Can you work these out from the model? Positions are in its coordinate system, mm. A direction names the side the tool comes from. Give positions to 0.01 mm unless a question says otherwise; leave off trailing zeros. Write each loop counter-clockwise with the first axis right and the second up, starting at its lowest first coordinate (ties: lowest second). Pieces come first, ordered by that corner, then holes.
from build123d import *

# Parameters (mm, degrees)
SKETCH_1_W          = 45
SKETCH_1_H          = 26
EXTRUDE_1_DEPTH     = 18
SKETCH_2_W          = 47
SKETCH_2_H          = 28
EXTRUDE_2_DEPTH     = 2
SKETCH_3_W          = 39
SKETCH_3_H          = 20
CUT_EXTRUDE_2_DEPTH = 2
CHAMFER_1_SIZE      = 2


with BuildPart() as part:
    # 草图1 → 凸台-拉伸1 (new body)
    with BuildSketch(Plane(origin=(0, 0, 0), x_dir=(1, 0, 0), z_dir=(0, 1, 0))):
        Rectangle(SKETCH_1_W, SKETCH_1_H)
    extrude(amount=EXTRUDE_1_DEPTH)

    # 草图2 → 凸台-拉伸2 (add)
    with BuildSketch(Plane(origin=(0, 18, 0), x_dir=(1, 0, 0), z_dir=(0, 1, 0))):
        Rectangle(SKETCH_2_W, SKETCH_2_H)
    extrude(amount=EXTRUDE_2_DEPTH)

    # 草图3 → 切除-拉伸2 (cut)
    with BuildSketch(Plane(origin=(0, 20, 0), x_dir=(1, 0, 0), z_dir=(0, 1, 0))):
        Rectangle(SKETCH_3_W, SKETCH_3_H)
    extrude(amount=-CUT_EXTRUDE_2_DEPTH, mode=Mode.SUBTRACT)

    # 倒角1
    chamfer_1_edges = [part.edges().sort_by_distance(p)[0] for p in [
        (-19.5, 20, 0),
        (0, 20, 10),
        (19.5, 20, 0),
        (0, 20, -10),
    ]]
    chamfer(chamfer_1_edges, length=CHAMFER_1_SIZE - 0.0001)  # a hair under: the kernel refuses the full size


solid = part.part
(1) Imagine slicing it at D-D, the plane z = 11. Write out the boundary of the cut face in (x, y).
Returned:
outline: (-23.5, 18) - (-22.5, 18) - (-22.5, 0) - (22.5, 0) - (22.5, 18) - (23.5, 18) - (23.5, 20) - (21.5, 20) - (20.5, 19) - (-20.5, 19) - (-21.5, 20) - (-23.5, 20) - close
(2) For faces 1 (the face through (20.5, 19, 0.2)), 2 (the face through (22.5, 9, 0)), 3 (the face through (0, 9, 13)), 4 (the face through (-22.5, 9, 0)), which set-ups out of +Z, -Z, +X, -X, +Y, -Y let a thin tool reach every point of the face, with its end or its side?
Returned:
face 1: +Y
face 2: +Z, -Z, +X, -Y
face 3: +Z, +X, -X, -Y
face 4: +Z, -Z, -X, -Y
(3) If we mould it in two halves opening along Z, with no side actions, what happens to faces 5 (the face through (-20.5, 19, 0.2)), 6 (the face through (0, 18, 0)), 7 (the face through (-23.5, 19, 0)), 8 (the face through (0, 9, -13))? For each: +Z half, -Z half, draft (parallel to the pull), parting line (faces both ways), or undercut.
Returned:
face 5: undercut
face 6: undercut
face 7: draft
face 8: -Z half
(4) Will these pins go through, and if not, where does the flat tip stop? P1, Ø12, axis at x = -0.5, z = 8.5, coming from the +Y side; P2, Ø1, axis at x = -9.5, y = 8.5, coming from the -Z side; P3, Ø2, axis at y = 15, z = -6, coming from the -X side; P4, Ø1.5, axis at x = 15, z = 3, coming from the +Y side.
Returned:
P1: stops at y = 20
P2: stops at z = -13
P3: stops at x = -22.5
P4: stops at y = 18
(5) Imagine slicing it at C-C, the plane y = 18.75. Write out the boundary of the cut face in (x, z).
Returned:
outline: (-23.5, -14) - (23.5, -14) - (23.5, 14) - (-23.5, 14) - close; hole (-20.25, -10.75) - (20.25, -10.75) - (20.25, 10.75) - (-20.25, 10.75) - close
(6) If I drill on L1, parallel to Z at x = -8.5, y = 6.5; L2, parallel to Y at x = 4, z = -6; L3, parallel to X at y = 2.75, z = -1.5, over which ranges is the centre line in solid material (lowest first)?
Returned:
L1: z = -13 to 13
L2: y = 0 to 18
L3: x = -22.5 to 22.5
